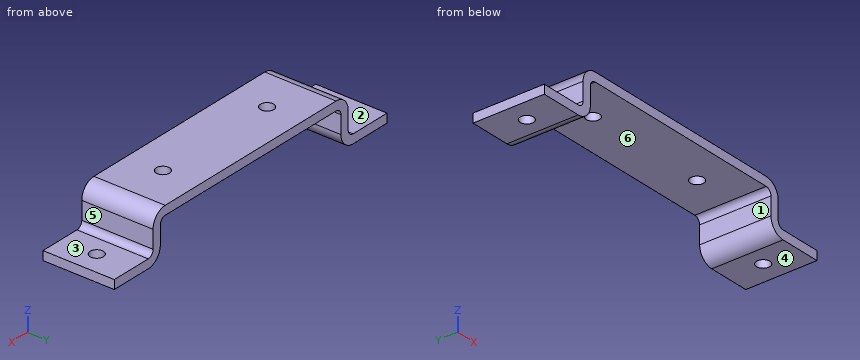
```python
from build123d import *

# Parameters (mm, degrees)
F1_DEPTH = 38.1
F2_R     = 6.35
F3_R     = 15.875
F4_R     = 7.14375
F5_DEPTH = 25.4
F6_R     = 7.14375
F7_DEPTH = 25.4


with BuildPart() as f1:
    # F0 (on Front) → F1 (new body, symmetric)
    with BuildSketch(Plane.XZ):
        Polygon((-178.59375, -15.875), (-178.59375, -25.4), (-118.26875, -25.4), (-118.26875, 15.875), (118.26875, 15.875), (118.26875, -25.4), (178.59375, -25.4), (178.59375, -15.875), (127.79375, -15.875), (127.79375, 25.4), (-127.79375, 25.4), (-127.79375, -15.875), align=None)
    extrude(amount=F1_DEPTH, both=True)

    # F2
    f2_edges = [f1.edges().sort_by_distance(p)[0] for p in [
        (-127.79375, 0, -15.875),
        (-118.26875, 0, 15.875),
        (118.26875, 0, 15.875),
        (127.79375, 0, -15.875),
    ]]
    fillet(f2_edges, radius=F2_R)

    # F3
    f3_edges = [f1.edges().sort_by_distance(p)[0] for p in [
        (-127.79375, 0, 25.4),
        (127.79375, 0, 25.4),
        (118.26875, 0, -25.4),
        (-118.26875, 0, -25.4),
    ]]
    fillet(f3_edges, radius=F3_R)

    # F4 (on face) → F5 (cut)
    with BuildSketch(Plane.XY.offset(25.4)):
        with Locations((-68.2625, 0)):
            Circle(F4_R)
        with Locations((68.2625, 0)):
            Circle(F4_R)
    extrude(amount=-F5_DEPTH, mode=Mode.SUBTRACT)

    # F6 (on face) → F7 (cut)
    with BuildSketch(Plane.XY.offset(-15.875)):
        with Locations((-154.78125, 0)):
            Circle(F6_R)
        with Locations((154.78125, 0)):
            Circle(F6_R)
    extrude(amount=-F7_DEPTH, mode=Mode.SUBTRACT)


solid = f1.part
```
Verification items for the finished model (mm, model axes). Face numbers are marked on the shaded views. A direction names the side the tool comes from. Round coordinates to 2 decimals unless told otherwise and drop trailing zeros. Order: outer loops, then holes, each group sorted by start corner. A loop starts at its lowest first (then second) coordinate and runs counter-clockwise, first axis right, second up. Notation, with made-up numbers: (44, 17) - (89, 17) arc R7 cw to (89, 25) - close; hole circle Ø3 at (-3, 4). An arc over 180 degrees is marked (long way). Use CSV: the item, a comma, the result in double quotes.
(1) Mould release check, pull along X, two halves, no side actions. Record for the marked faces 4, 5 and 6: released by +X, released by -X, zero draft, split by the parting line, or undercut.
Entries:
face 4,"zero draft"
face 5,"released by +X"
face 6,"undercut"
(2) Gauge pin test, flat ends, axial feed: pin 1 Ø2 at (y, z) = (-24.5, 1) entering from -X; pin 2 Ø8 at (y, z) = (-22.5, -6.5) entering from +X; pin 3 Ø8.5 at (x, y) = (-68.26, 0) entering from -Z; pin 4 Ø5 at (y, z) = (-2, 16.5) entering from -X. Record the tip position at first contact, or that the pin passes through.
Entries:
pin 1,"x = -127.79"
pin 2,"x = 127.87"
pin 3,"through"
pin 4,"x = -127.15"
(3) Thickness scan on probe 1 along X at (y, z) = (14.5, -5); probe 2 along X at (y, z) = (4.5, 16.5); probe 3 along Z at (x, y) = (81, -16.5) (3 decimals). Record the ranges inside material, lowest first. Write a range as from..to.
Entries:
probe 1,"-127.79..-118.27, 118.27..127.79"
probe 2,"-126.18..-73.81, -62.71..62.71, 73.81..126.18"
probe 3,"15.875..25.4"
(4) Section check A-A on z = 2.5. Record the boundary of the cut face in (x, y), and give its area (3 significant figures).
Entries:
outline,"(-127.79, -38.1) - (-118.27, -38.1) - (-118.27, 38.1) - (-127.79, 38.1) - close; (118.27, -38.1) - (127.79, -38.1) - (127.79, 38.1) - (118.27, 38.1) - close"
area,"1,450 mm^2"
(5) Section check C-C on y = -32.5. Record the boundary of the cut face in (x, z) (3 decimals).
Entries:
outline,"(-178.594, -25.4) - (-134.144, -25.4) arc R15.875 ccw to (-118.269, -9.525) - (-118.269, 9.525) arc R6.35 cw to (-111.919, 15.875) - (111.919, 15.875) arc R6.35 cw to (118.269, 9.525) - (118.269, -9.525) arc R15.875 ccw to (134.144, -25.4) - (178.594, -25.4) - (178.594, -15.875) - (134.144, -15.875) arc R6.35 cw to (127.794, -9.525) - (127.794, 9.525) arc R15.875 ccw to (111.919, 25.4) - (-111.919, 25.4) arc R15.875 ccw to (-127.794, 9.525) - (-127.794, -9.525) arc R6.35 cw to (-134.144, -15.875) - (-178.594, -15.875) - close"
(6) Access from +Z, -Z, +X, -X, +Y, -Y to the whole of each face (thin tool, end or side, straight path). Record for the marked faces 1, 2 and 3.
Entries:
face 1,"-Z, +Y, -Y"
face 2,"+Z, -X, +Y, -Y"
face 3,"+Z, +X, +Y, -Y"
(7) Section check B-B on x = 71.5. Record the boundary of the cut face in (y, z) (3 decimals).
Entries:
outline,"(-38.1, 15.875) - (-6.368, 15.875) - (-6.368, 25.4) - (-38.1, 25.4) - close; (6.368, 15.875) - (38.1, 15.875) - (38.1, 25.4) - (6.368, 25.4) - close"
(8) Section check D-D on y = 0. State how many separate pieces and enclosed holes the cut face has, and give its area (3 significant figures).
Entries:
separate pieces,"5"
enclosed holes,"0"
area,"3,460 mm^2"
